Job drawing, mm, ordinate dimensions from the low corner. One solid piece. Coordinates: 2 decimals unless noted, no trailing zeros. Loops run counter-clockwise (first coordinate to the right, second up) from the corner with the lowest first, then second, coordinate; pieces in that order, holes last. Notation, with made-up numbers: M 83,80 L 141,80 A30 cw 141,116 Z; hole C -38.5,71.5 d7. An arc over 180 degrees is marked long. Answer as a JSON object with one key per item and string values. Group by question number.
1. Drill centre lines: L1, parallel to X at y = 2.2, z = 15; L2, parallel to Z at x = 53, y = 0.25. Where is each one in solid material? Low to high.
2. Saw through at D-D on y = 1.15. Write the cut outline in (x, z).
3. Saw through at B-B on x = 185. Write the cut outline in (y, z), then the cut area to 3 significant figures.
4. Drop a flat-ended pin along its axis: pin 1 Ø3 at (x, z) = (15, 15) entering from +Y. Give the stop position or say it passes through.
5. Saw through at A-A on z = 60. Write the cut outline in (x, y), then the cut area to 3 significant figures.
6. Saw through at C-C on x = 125.5. Write the cut outline in (y, z).
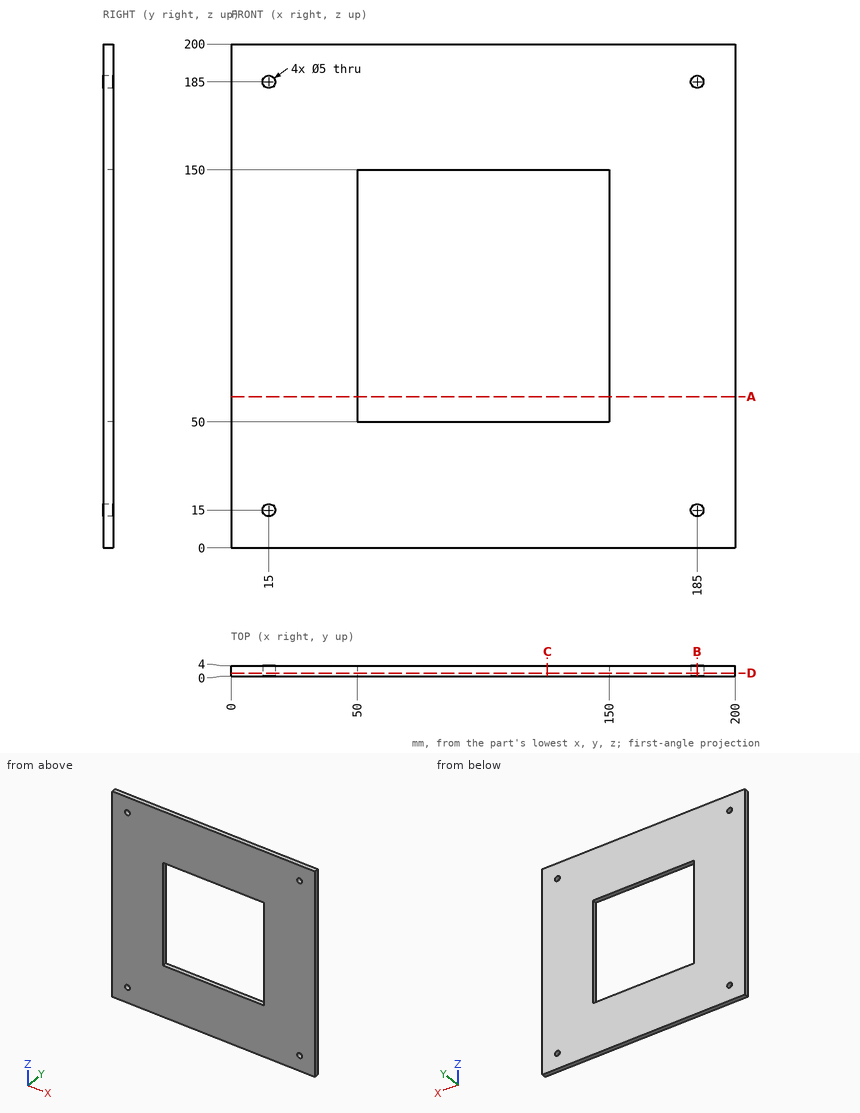
Outcome:
{
 "1": {"L1": "x = 0 to 12.5, 17.5 to 182.5, 187.5 to 200", "L2": "z = 0 to 50, 150 to 200"},
 "2": {"outline": "M 0,0 L 200,0 L 200,200 L 0,200 Z; hole C 15,15 d5; hole C 15,185 d5; hole M 50,50 L 150,50 L 150,150 L 50,150 Z; hole C 185,15 d5; hole C 185,185 d5"},
 "3": {"outline": "M 0,0 L 4,0 L 4,12.5 L 0,12.5 Z; M 0,17.5 L 4,17.5 L 4,182.5 L 0,182.5 Z; M 0,187.5 L 4,187.5 L 4,200 L 0,200 Z", "area": "760 mm²"},
 "4": {"pin 1": "passes through"},
 "5": {"outline": "M 0,0 L 50,0 L 50,4 L 0,4 Z; M 150,0 L 200,0 L 200,4 L 150,4 Z", "area": "400 mm²"},
 "6": {"outline": "M 0,0 L 4,0 L 4,50 L 0,50 Z; M 0,150 L 4,150 L 4,200 L 0,200 Z"}
}
